Read the model definition and answer for the solid it produces. Units are mm, in the model's axes. Coordinates: 2 decimals unless noted, no trailing zeros. Write each loop counter-clockwise with the first axis right and the second up, starting at its lowest first coordinate (ties: lowest second). Pieces come first, ordered by that corner, then holes. Notation, with made-up numbers: (-35.5, 57) -> (-27.5, 57) arc R18 ccw to (-27.5, 89) -> close; hole circle Ø2 at (3, 65). An arc over 180 degrees is marked (long way). Use CSV: the item, a comma, the result in double quotes.
from build123d import *

# Parameters (mm, degrees)
BOSS_EXTRUDE1_DEPTH = 12.7
SKETCH2_R           = 2.1828125
CUT_EXTRUDE1_DEPTH  = 62.362637457


with BuildPart() as part:
    # Sketch1 → Boss-Extrude1 (new body)
    with BuildSketch(Plane.XY):
        with BuildLine():
            Line((-31.9913, 0), (-19.2913, 0))
            ThreePointArc((-19.2913, 0), (0, -19.2913), (19.2913, 0))
            Line((19.2913, 0), (31.9913, 0))
            Line((31.9913, 0), (31.9913, -50.8))
            Line((31.9913, -50.8), (-31.9913, -50.8))
            Line((-31.9913, -50.8), (-31.9913, 0))
        make_face()
    extrude(amount=BOSS_EXTRUDE1_DEPTH)

    # Sketch2 → Cut-Extrude1 (cut, through all)
    with BuildSketch(Plane.XZ.offset(50.8)):
        with Locations((-25.6413, 6.35)):
            Circle(SKETCH2_R)
        with Locations((25.6413, 6.35)):
            Circle(SKETCH2_R)
    extrude(amount=-CUT_EXTRUDE1_DEPTH, mode=Mode.SUBTRACT)


solid = part.part
1. A cutting plane is placed at D-D (x = 0). Give the vertices of the cut face in (y, z), and give its area (3 significant figures).
Solutions:
outline,"(-50.8, 0) -> (-19.29, 0) -> (-19.29, 12.7) -> (-50.8, 12.7) -> close"
area,"400 mm^2"
2. A cutting plane is placed at B-B (y = -12.5). Give the vertices of the cut face in (x, z).
Solutions:
outline,"(-31.99, 0) -> (-14.69, 0) -> (-14.69, 12.7) -> (-31.99, 12.7) -> close; (14.69, 0) -> (31.99, 0) -> (31.99, 12.7) -> (14.69, 12.7) -> close; hole circle Ø4.37 at (-25.64, 6.35); hole circle Ø4.37 at (25.64, 6.35)"
3. This flat-tipped pin is pushed along its axis until it touches: pin 1 Ø4 at (x, z) = (-5.5, 3.5) entering from +Y. Where does it stop, or does it pass through?
Solutions:
pin 1,"stops at y = -17.77"
4. A cutting plane is placed at C-C (y = -31.5). Give the vertices of the cut face in (x, z).
Solutions:
outline,"(-31.99, 0) -> (31.99, 0) -> (31.99, 12.7) -> (-31.99, 12.7) -> close; hole circle Ø4.37 at (-25.64, 6.35); hole circle Ø4.37 at (25.64, 6.35)"
5. For a pull along X with two mould halves and no side action, classify faces 1 (the cylindrical face through (-0.424, -19.287, 6.261)), 2 (the flat face through (31.991, -25, 6)), 3 (the flat face through (-31.991, -26, 6)), 4 (the flat face through (-29, 0, 6)) as pulls with the +X half, pulls with the -X half, needs draft (parallel to the pull), parting line crosses it, or undercut.
Solutions:
face 1,"undercut"
face 2,"pulls with the +X half"
face 3,"pulls with the -X half"
face 4,"needs draft"
6. A cutting plane is placed at A-A (z = 6.35). Give the vertices of the cut face in (x, y), and give its area (3 significant figures).
Solutions:
outline,"(-31.99, -50.8) -> (-27.82, -50.8) -> (-27.82, 0) -> (-31.99, 0) -> close; (-23.46, -50.8) -> (23.46, -50.8) -> (23.46, 0) -> (19.29, 0) arc R19.29 cw to (-19.29, 0) -> (-23.46, 0) -> close; (27.82, -50.8) -> (31.99, -50.8) -> (31.99, 0) -> (27.82, 0) -> close"
area,"2,220 mm^2"
7. Find the intervals of material crossed by line 1 along X through (y, z) = (-28, 6.5); line 2 along X through (y, z) = (-39.5, 8.25); line 3 along X through (y, z) = (-16, 7.25), in increasing order.
Solutions:
line 1,"x = -31.99 to -27.82, -23.46 to 23.46, 27.82 to 31.99"
line 2,"x = -31.99 to -26.72, -24.57 to 24.57, 26.72 to 31.99"
line 3,"x = -31.99 to -27.63, -23.65 to -10.78, 10.78 to 23.65, 27.63 to 31.99"
